Work out the finished part from the listing and answer in its coordinate system (mm). Round coordinates to 2 decimals unless told otherwise and drop trailing zeros. Order: outer loops, then holes, each group sorted by start corner. A loop starts at its lowest first (then second) coordinate and runs counter-clockwise, first axis right, second up. Notation, with made-up numbers: (88, -21) -> (106, -21) arc R28 ccw to (106, 7) -> close; hole circle Ø5 at (-27, -21.5). An arc over 180 degrees is marked (long way). Use one line per item in the form item = value.
```python
from build123d import *

# Parameters (mm, degrees)
CROQUIS1_R              = 10
CROQUIS1_R_2            = 6.35
SALIENTE_EXTRUIR1_DEPTH = 7.9375


with BuildPart() as part:
    # Croquis1 → Saliente-Extruir1 (new body)
    with BuildSketch(Plane(origin=(0, 0, 0), x_dir=(0, 0, -1), z_dir=(1, 0, 0))):
        with BuildLine():
            Line((0, -35), (140, -35))
            Line((140, -35), (140, 35))
            Line((140, 35), (0, 35))
            ThreePointArc((0, 35), (-35, 0), (0, -35))
        make_face()
        Circle(CROQUIS1_R, mode=Mode.SUBTRACT)
        with Locations((65, 0)):
            Circle(CROQUIS1_R_2, mode=Mode.SUBTRACT)
        with Locations((125, 0)):
            Circle(CROQUIS1_R_2, mode=Mode.SUBTRACT)
    extrude(amount=SALIENTE_EXTRUIR1_DEPTH)


solid = part.part
```
Item 1: The part is cut by section A-A, the plane y = 0. Give the vertices of the cut face in (x, z).
Findings:
outline = (0, -140) -> (7.94, -140) -> (7.94, -131.35) -> (0, -131.35) -> close; (0, -118.65) -> (7.94, -118.65) -> (7.94, -71.35) -> (0, -71.35) -> close; (0, -58.65) -> (7.94, -58.65) -> (7.94, -10) -> (0, -10) -> close; (0, 10) -> (7.94, 10) -> (7.94, 35) -> (0, 35) -> close
Item 2: The part is cut by section D-D, the plane z = -4. Give the vertices of the cut face in (x, y).
Findings:
outline = (0, -35) -> (7.94, -35) -> (7.94, -9.17) -> (0, -9.17) -> close; (0, 9.17) -> (7.94, 9.17) -> (7.94, 35) -> (0, 35) -> close
Item 3: The part is cut by section B-B, the plane z = -65. Give the vertices of the cut face in (x, y), and give its area (3 significant figures).
Findings:
outline = (0, -35) -> (7.94, -35) -> (7.94, -6.35) -> (0, -6.35) -> close; (0, 6.35) -> (7.94, 6.35) -> (7.94, 35) -> (0, 35) -> close
area = 455 mm^2
Item 4: Consider line 1 along Y through (x, z) = (4.5, -125); line 2 along Z through (x, y) = (5.25, 2); line 3 along Z through (x, y) = (5.5, -30.5). Determine where each line is inside the solid, lowest interval first.
Findings:
line_1 = -35 to -6.35, 6.35 to 35
line_2 = -140 to -131.03, -118.97 to -71.03, -58.97 to -9.8, 9.8 to 34.94
line_3 = -140 to 17.17
Item 5: Flat-ended cylindrical pins translate along their axes: P1, Ø1, axis at x = 1, y = 2.5, coming from the +Z side; P2, Ø4, axis at x = 2.5, y = -3, coming from the +Z side; P3, Ø12, axis at y = 0, z = 0, coming from the +X side; P4, Ø3, axis at x = 5.5, y = 26, coming from the +Z side (3 decimals). Find the tip coordinate at first contact, or state that the pin passes through.
Findings:
P1 = 34.94
P2 = 34.99
P3 = through
P4 = 24.995
Item 6: The part is cut by section C-C, the plane x = 6.25. Give the vertices of the cut face in (y, z), and give its area (3 significant figures).
Findings:
outline = (-35, -140) -> (35, -140) -> (35, 0) arc R35 ccw to (-35, 0) -> close; hole circle Ø20 at (0, 0); hole circle Ø12.7 at (0, -125); hole circle Ø12.7 at (0, -65)
area = 11,200 mm^2
Item 7: Determine the mould class of faces 1 (the flat face through (4, 35, -71)), 2 (the cylindrical face through (3.913, 0.279, -58.656)), 3 (the flat face through (0, 0, -51)), 4 (the cylindrical face through (3.91, -9.76, 2.17)) for opening direction Y: released by +Y, released by -Y, zero draft, split by the parting line, or undercut.
Findings:
face_1 = released by +Y
face_2 = undercut
face_3 = zero draft
face_4 = undercut
